```python
from build123d import *

# Parameters (mm, degrees)
F5_DEPTH      = 5
F3_R          = 30
F6_DEPTH      = 12.5
F7_COUNT      = 6
F8_R          = 30
F8_R_2        = 15
F9_DEPTH      = 8.3
F9_DEPTH_BACK = 8.3


with BuildPart() as f5:
    # F2 (on line) → F5 (new body, symmetric)
    with BuildSketch(Plane(origin=(0, 0, 0), x_dir=(1, 0, 0), z_dir=(0, 0.5, -0.8660254038))):
        with BuildLine():
            Line((28.9777747887, -7.7645713531), (96.5925826289, -25.8819045103))
            ThreePointArc((96.5925826289, -25.8819045103), (100, 0), (96.5925826289, 25.8819045103))
            Line((96.5925826289, 25.8819045103), (28.9777747887, 7.7645713531))
            Line((28.9777747887, 7.7645713531), (0, 0))
            Line((0, 0), (28.9777747887, -7.7645713531))
        make_face()
    extrude(amount=F5_DEPTH, both=True)

    # F3 (on Top) → F6 (cut, symmetric)
    with BuildSketch(Plane.XY):
        Circle(F3_R)
    extrude(amount=F6_DEPTH, both=True, mode=Mode.SUBTRACT)


with BuildPart() as f7_1:
    # F7: instance of F5
    add(f5.part.rotate(Axis((0, 0, 1.348067075), (0, 0, 1)), 1 * 360 / F7_COUNT))


with BuildPart() as f7_2:
    # F7: instance of F5
    add(f5.part.rotate(Axis((0, 0, 1.348067075), (0, 0, 1)), 2 * 360 / F7_COUNT))


with BuildPart() as f7_3:
    # F7: instance of F5
    add(f5.part.rotate(Axis((0, 0, 1.348067075), (0, 0, 1)), 3 * 360 / F7_COUNT))


with BuildPart() as f7_4:
    # F7: instance of F5
    add(f5.part.rotate(Axis((0, 0, 1.348067075), (0, 0, 1)), 4 * 360 / F7_COUNT))


with BuildPart() as f7_5:
    # F7: instance of F5
    add(f5.part.rotate(Axis((0, 0, 1.348067075), (0, 0, 1)), 5 * 360 / F7_COUNT))


with BuildPart() as f5_1:
    add(f5.part)

    add(f7_1.part)  # F9 merges F7_1

    add(f7_2.part)  # F9 merges F7_2

    add(f7_3.part)  # F9 merges F7_3

    add(f7_4.part)  # F9 merges F7_4

    add(f7_5.part)  # F9 merges F7_5
    # F8 (on Top) → F9 (join, two sides)
    with BuildSketch(Plane.XY) as f9_sk:
        Circle(F8_R)
        Circle(F8_R_2, mode=Mode.SUBTRACT)
    extrude(amount=F9_DEPTH)
    extrude(f9_sk.sketch, amount=-F9_DEPTH_BACK)


solid = f5_1.part
```
Verification items for the finished model (mm, model axes). A direction names the side the tool comes from. Give positions to 0.01 mm unless a question says otherwise; leave off trailing zeros. Order: outer loops, then holes, each group sorted by start corner. A loop starts at its lowest first (then second) coordinate and runs counter-clockwise, first axis right, second up. Notation, with made-up numbers: (-0.75, -31.5) - (17.25, -31.5) arc R25 cw to (17.25, 0.5) - close; hole circle Ø9 at (-26, 85.25). An arc over 180 degrees is marked (long way). Answer as CSV lines item,"result". Start each with the question number.
Item 1: Mould release check, pull along X, two halves, no side actions. Record for faces 1 (the face through (62.11, 14.45, 8.26)), 2 (the face through (44.17, 47.31, -8.51)), 3 (the face through (-50.3, 86.43, 0.12)): released by +X, released by -X, zero draft, split by the parting line, or undercut.
Item 2: Section check D-D, the plane x = -73. Record the boundary of the cut face in (y, z).
Item 3: Material ranges on L1, parallel to Y at x = 0, z = 4.75; L2, parallel to X at y = 2, z = -8; L3, parallel to Z at x = 37, y = 46, recorded low to high.
Item 4: Section check A-A, the plane x = 0. Record the boundary of the cut face in (y, z), plus the area to 3 significant figures.
Item 5: Section check C-C, the plane z = 12.5. State how many separate pieces and enclosed holes the cut face has, plus the area to 3 significant figures.
Item 6: Access from +Z, -Z, +X, -X, +Y, -Y to the whole of each face (thin tool, end or side, straight path). Record for faces 4 (the face through (-37.76, 61.02, -4.51)), 5 (the face through (38.3, 60.71, 4.15)), 6 (the face through (-26.12, -14.76, 0.12)), 7 (the face through (-63.061, 14.598, -8.509)).
Item 7: Section check B-B, the plane y = 58. Record the boundary of the cut face in (x, z).
Item 8: Gauge pin test, flat ends, axial feed: pin 1 (1 mm diameter, centred on y = 58, z = 2, fed in from +X); pin 2 (1 mm diameter, centred on y = -16.5, z = -3, fed in from +X); pin 3 (10 mm diameter, centred on y = 55, z = 7, fed in from +X). Record the tip position at first contact, or that the pin passes through.
Filled in:
1,face 1,"undercut"
1,face 2,"released by +X"
1,face 3,"released by -X"
2,outline,"(-19.44, 5.45) - (14.44, -14.11) - (19.44, -5.45) - (-14.44, 14.11) - close"
3,L1,"-30 to -15, 15 to 30"
3,L2,"-29.93 to -14.87, 14.87 to 29.93"
3,L3,"-10.99 to 0.55"
4,outline,"(-30, -8.3) - (-15, -8.3) - (-15, 8.3) - (-30, 8.3) - close; (15, -8.3) - (30, -8.3) - (30, 8.3) - (15, 8.3) - close"
4,area,"498 mm^2"
5,separate pieces,"6"
5,enclosed holes,"0"
5,area,"1,250 mm^2"
6,face 4,"-Z, -X"
6,face 5,"+Z, +X"
6,face 6,"none"
6,face 7,"-Z"
7,outline,"(-57.54, 6.25) - (-20.21, -12.41) - (-15.12, -3.41) - (-50.87, 14.47) - close; (15.12, 3.41) - (50.87, -14.47) - (57.54, -6.25) - (20.21, 12.41) - close"
8,pin 1,"x = 42.07"
8,pin 2,"x = 25.38"
8,pin 3,"x = 39.71"
